Read the model definition and answer for the solid it produces. Units are mm, in the model's axes. Face numbers are marked on the shaded views. A direction names the side the tool comes from. Give positions to 0.01 mm unless a question says otherwise; leave off trailing zeros. Loops run counter-clockwise (first coordinate to the right, second up) from the corner with the lowest first, then second, coordinate; pieces in that order, holes last. Notation, with made-up numbers: (-11.75, -5.5) -> (17.25, -5.5) arc R20 cw to (17.25, 0.5) -> close; hole circle Ø8 at (-38, -4.5). An arc over 180 degrees is marked (long way). Answer as CSV lines item,"result". Start each with the question number.
```python
from build123d import *

# Parameters (mm, degrees)
SKETCH_1_W      = 29
SKETCH_1_H      = 2.5
SKETCH_2_R      = 1
EXTRUDE_1_DEPTH = 20


with BuildPart() as part:
    # 草图1 → 旋转1 (revolve)
    with BuildSketch(Plane.XY):
        with BuildLine():
            add(Edge.make_bspline(
                [(-14.25, 20.5), (-10.271097928, 9.254557994), (-6.75, 21)],
                knots=[0, 0, 0, 1, 1, 1], degree=2))
            Line((-6.75, 21), (-6.75, 29.5))
            Line((-6.75, 29.5), (0, 29.5))
            Line((0, 29.5), (0, 0))
            Line((0, 0), (-21, 0))
            Line((-21, 0), (-21, 29.5))
            Line((-21, 29.5), (-14.25, 29.5))
            Line((-14.25, 29.5), (-14.25, 20.5))
        make_face()
        with Locations((14.5, 1.25)):
            Rectangle(SKETCH_1_W, SKETCH_1_H)
    revolve(axis=Axis((0, 0, 0), (-1, 0, 0)))

    # 草图2 → 凸台-拉伸1 (add)
    with BuildSketch(Plane(origin=(0, 0, 0), x_dir=(0, 0, -1), z_dir=(1, 0, 0))):
        with Locations(Location((0, 22.5, 0), (0, 0, 270))):
            Circle(SKETCH_2_R)
        with Locations(Location((0, -22.5, 0), (0, 0, 270))):
            Circle(SKETCH_2_R)
    extrude(amount=-EXTRUDE_1_DEPTH)


solid = part.part
```
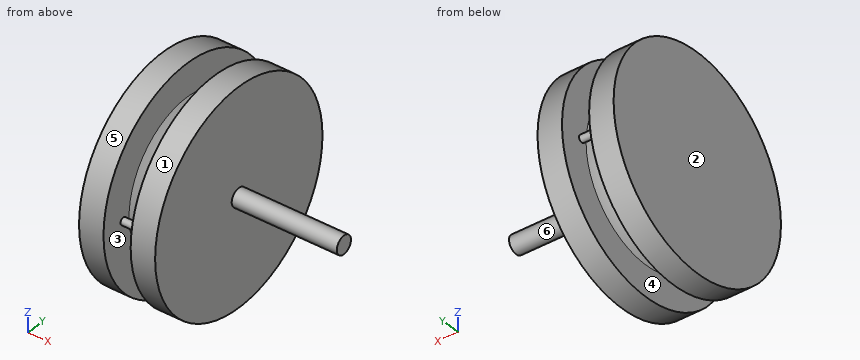
(1) Find section B-B on z = 23.5. Write down the section's boundary in (x, y).
(2) The mould has two halves that part along X. Classify the marked faces 1, 2 and 3: pulls with the +X half, pulls with the -X half, needs draft (parallel to the pull), parting line crosses it, or undercut.
(3) Find section C-C on z = 0. Give the number of separate pieces and of enclosed holes in the cut face, then the cut area to 3 significant figures.
(4) Find section D-D on y = 22.5. Write down the section's boundary in (x, z), then the cut area to 3 significant figures.
(5) Find the intervals of material crossed by line 1 along X through (y, z) = (26, -5); line 2 along X through (y, z) = (-17, 6.5); line 3 along X through (y, z) = (-9, 11), in increasing order. Write a range as from..to.
(6) Find section A-A on y = -24.5. Write down the section's boundary in (x, z), then the cut area to 3 significant figures.
(7) Each of these flat-tipped pins is pushed along its axis until it touches: P1, Ø8, axis at x = 0, y = -9.5, coming from the -Z side; P2, Ø12, axis at y = 12, z = 17, coming from the +X side; P3, Ø12, axis at x = -13, z = -22.5, coming from the +Y side. Where does it stop, or does it pass through?
(8) A tool of negligible diameter and unlimited length cuts with its end or side. For the marked faces 4, 5 and 6, from which of +Z, -Z, +X, -X, +Y, -Y can it reach the whole face along a straight path? Write none if from no direction.
Answer block:
1,outline,"(-21, -17.83) -> (-14.25, -17.83) -> (-14.25, 17.83) -> (-21, 17.83) -> close; (-6.75, -17.83) -> (0, -17.83) -> (0, 17.83) -> (-6.75, 17.83) -> close"
2,face 1,"needs draft"
2,face 2,"pulls with the -X half"
2,face 3,"undercut"
3,separate pieces,"1"
3,enclosed holes,"2"
3,area,"1,230 mm2"
4,outline,"(-21, -19.08) -> (-14.25, -19.08) -> (-14.25, -1) -> (-6.75, -1) -> (-6.75, -19.08) -> (0, -19.08) -> (0, 19.08) -> (-6.75, 19.08) -> (-6.75, 1) -> (-14.25, 1) -> (-14.25, 19.08) -> (-21, 19.08) -> close"
4,area,"530 mm2"
5,line 1,"x = -21..-14.25, -6.75..0"
5,line 2,"x = -21..-13.33, -7.73..0"
5,line 3,"x = -21..0"
6,outline,"(-21, -16.43) -> (-14.25, -16.43) -> (-14.25, 16.43) -> (-21, 16.43) -> close; (-6.75, -16.43) -> (0, -16.43) -> (0, 16.43) -> (-6.75, 16.43) -> close"
6,area,"444 mm2"
7,P1,"stops at z = -28.98"
7,P2,"stops at x = 0"
7,P3,"stops at y = 24.36"
8,face 4,"none"
8,face 5,"+X, -X"
8,face 6,"+X"
